Could you check a few things on this model? Use its own coordinates, in mm. A direction names the side the tool comes from. Give positions to 0.01 mm unless a question says otherwise; leave off trailing zeros. Loops run counter-clockwise (first coordinate to the right, second up) from the corner with the lowest first, then second, coordinate; pieces in that order, holes last. Notation, with made-up numbers: M 14,84 L 51,84 A16 ccw 51,108 Z; hole C 12.25,-34 d3. An arc over 180 degrees is marked long. Answer in a Markdown table with one row per item. Add a question column.
1. If we section it at D-D on y = 6: List the corners of the cut face in (x, z) for me.
2. If we section it at A-A on x = 1.75: List the corners of the cut face in (y, z) for me, then the cut area to 4 significant figures.
3. If we section it at B-B on z = -10.5: List the corners of the cut face in (x, y) for me, then the cut area to 4 significant figures.
4. Thinking about a two-plate mould opening in X: for faces 1 (the flat face through (-40.5, 10, 1)), 2 (the flat face through (-1, 0, 21)), 3 (the cylindrical face through (1.86, 8.619, 19.502)), which applies, released by +X, released by -X, zero draft, split by the parting line, or undercut?
5. I'm going to push a flat-ended pin straight in: pin 1 Ø1.5 at (x, z) = (22, 10) entering from +Y. Where does the tip first touch, or does it pass through?
6. If we section it at C-C on x = 34.25: List the corners of the cut face in (y, z) for me, then the cut area to 3 significant figures.
7. I need wall thicknesses on line 1 along X through (y, z) = (8, -10.5); line 2 along Z through (x, y) = (-31, 11); line 3 along X through (y, z) = (12, -43). Which ranges of each line are inside material? Lowest first, please. Write a range as from..to.
8. Which directions (+Z, -Z, +X, -X, +Y, -Y) give clear straight access to the entire face, cutting with the end or side of a thin tool? Please do faces 4 (the flat face through (1, 19, -47.5)), 5 (the flat face through (-6, 20, 29)).
```python
from build123d import *

# Parameters (mm, degrees)
SKETCH1_W           = 81
SKETCH1_H           = 97
BOSS_EXTRUDE1_DEPTH = 20
SKETCH2_R           = 28.25
CUT_EXTRUDE2_DEPTH  = 67.275938319
SKETCH5_W           = 74
SKETCH5_H           = 74
CUT_EXTRUDE3_DEPTH  = 3
SKETCH6_R           = 2.5
CUT_EXTRUDE4_DEPTH  = 66.433172015


with BuildPart() as part:
    # Sketch1 → Boss-Extrude1 (new body)
    with BuildSketch(Plane(origin=(0, 0, 0), x_dir=(1, 0, 0), z_dir=(0, 1, 0))):
        Rectangle(SKETCH1_W, SKETCH1_H)
    extrude(amount=BOSS_EXTRUDE1_DEPTH)

    # Sketch2 → Cut-Extrude2 (cut, through all)
    with BuildSketch(Plane(origin=(0, 20, 0), x_dir=(1, 0, 0), z_dir=(0, 1, 0))):
        with Locations(Location((1.75, 10.5, 0), (0, 0, 270))):
            Circle(SKETCH2_R)
    extrude(amount=-CUT_EXTRUDE2_DEPTH, mode=Mode.SUBTRACT)

    # Sketch5 → Cut-Extrude3 (cut)
    with BuildSketch(Plane(origin=(0, 20, 0), x_dir=(1, 0, 0), z_dir=(0, 1, 0))):
        with Locations((1.75, 10.5)):
            Rectangle(SKETCH5_W, SKETCH5_H)
    extrude(amount=-CUT_EXTRUDE3_DEPTH, mode=Mode.SUBTRACT)

    # Sketch6 → Cut-Extrude4 (cut, through all)
    with BuildSketch(Plane(origin=(0, 17, 0), x_dir=(1, 0, 0), z_dir=(0, 1, 0))):
        with Locations(Location((-30.75, 10.5, 0), (0, 0, 270))):
            Circle(SKETCH6_R)
        with Locations(Location((1.75, -22, 0), (0, 0, 270))):
            Circle(SKETCH6_R)
        with Locations(Location((34.25, 10.5, 0), (0, 0, 270))):
            Circle(SKETCH6_R)
        with Locations(Location((1.75, 43, 0), (0, 0, 270))):
            Circle(SKETCH6_R)
    extrude(amount=-CUT_EXTRUDE4_DEPTH, mode=Mode.SUBTRACT)


solid = part.part
```
Results:
| question | item | result |
|---|---|---|
| 1 | outline | M -40.5,-48.5 L 40.5,-48.5 L 40.5,48.5 L -40.5,48.5 Z; hole C -30.75,-10.5 d5; hole C 1.75,-10.5 d56.5; hole C 1.75,-43 d5; hole C 1.75,22 d5; hole C 34.25,-10.5 d5 |
| 2 | outline | M 0,-48.5 L 20,-48.5 L 20,-47.5 L 17,-47.5 L 17,-45.5 L 0,-45.5 Z; M 0,-40.5 L 17,-40.5 L 17,-38.75 L 0,-38.75 Z; M 0,17.75 L 17,17.75 L 17,19.5 L 0,19.5 Z; M 0,24.5 L 17,24.5 L 17,26.5 L 20,26.5 L 20,48.5 L 0,48.5 Z |
| 2 | area | 587.5 mm2 |
| 3 | outline | M -40.5,0 L -33.25,0 L -33.25,17 L -35.25,17 L -35.25,20 L -40.5,20 Z; M -28.25,0 L -26.5,0 L -26.5,17 L -28.25,17 Z; M 30,0 L 31.75,0 L 31.75,17 L 30,17 Z; M 36.75,0 L 40.5,0 L 40.5,20 L 38.75,20 L 38.75,17 L 36.75,17 Z |
| 3 | area | 267.5 mm2 |
| 4 | face 1 | released by -X |
| 4 | face 2 | zero draft |
| 4 | face 3 | undercut |
| 5 | pin 1 | y = 17 |
| 6 | outline | M 0,-48.5 L 20,-48.5 L 20,-47.5 L 17,-47.5 L 17,-13 L 0,-13 Z; M 0,-8 L 17,-8 L 17,26.5 L 20,26.5 L 20,48.5 L 0,48.5 Z |
| 6 | area | 1,630 mm2 |
| 7 | line 1 | -40.5..-33.25, -28.25..-26.5, 30..31.75, 36.75..40.5 |
| 7 | line 2 | -48.5..-12.99, -8.01..48.5 |
| 7 | line 3 | -40.5..-0.75, 4.25..40.5 |
| 8 | face 4 | +Y |
| 8 | face 5 | +Z, -Z, +X, -X, +Y |
